Design review of the part built by this model. Coordinates are the model's own, in mm. A direction names the side the tool comes from. Give positions to 0.01 mm unless a question says otherwise; leave off trailing zeros. Loops run counter-clockwise (first coordinate to the right, second up) from the corner with the lowest first, then second, coordinate; pieces in that order, holes last. Notation, with made-up numbers: (58, 44) -> (105, 44) arc R21 cw to (105, 65) -> close; hole circle Ø8 at (-21.5, -21). An arc over 180 degrees is marked (long way). Answer in a Markdown table with one row per item. Add a question column.
(1) Consider section A-A on y = -2.55. Write out the cut boundary in (x, z), then the cut area to 3 significant figures.
(2) Consider section D-D on x = 4.75. Write out the cut boundary in (y, z), then the cut area to 3 significant figures.
(3) Consider section B-B on x = 2.75. Write out the cut boundary in (y, z), then the cut area to 3 significant figures.
(4) Draft analysis for pull direction X (two halves, no side actions). For faces 1 (the cylindrical face through (3.23, -2.339, 6.393)), 2 (the cylindrical face through (5.45, -1.2, 5.58)), 3 (the flat face through (3, -3.15, 1)), 4 (the flat face through (4, -2, 1.55)), state which applies: +X half, -X half, draft (parallel to the pull), parting line (faces both ways), or undercut.
(5) For line 1 (Y direction, x = 5, z = 4.5); line 2 (X direction, y = -1.6, z = 5), list the stretches that pass through material, from the lowest coordinate up.
(6) For faces 5 (the flat face through (0, -2, 4)), 6 (the flat face through (4, -1.55, 4)), list the 3-axis set-ups (+Z, -Z, +X, -X, +Y, -Y) from which the entire face can be reached by the end or side of a thin tool; tool diameter is ignored.
(7) Consider section C-C on z = 3. Write out the cut boundary in (x, y), then the cut area to 3 significant figures.
(8) For pin 1 (0.8 mm diameter, centred on x = 3, y = -2, fed in from +Z); pin 2 (0.5 mm diameter, centred on y = -2.5, z = 3, fed in from +X), all flat-tipped, find the tip position at first contact; note any pin that passes through.
from build123d import *

# Parameters (mm, degrees)
BOSS_EXTRUDE1_DEPTH = 3.15
SHELL1_T            = -1.55
SKETCH2_R           = 2.440449026
CUT_EXTRUDE1_DEPTH  = 1.6


with BuildPart() as part:
    # Sketch1 → Boss-Extrude1 (new body)
    with BuildSketch(Plane(origin=(0, 0, 0), x_dir=(1, 0, 0), z_dir=(0, 1, 0))):
        with BuildLine():
            Line((0, 0), (0, -7.8))
            ThreePointArc((0, -7.8), (5.515432893, -5.515432893), (7.8, 0))
            Line((7.8, 0), (0, 0))
        make_face()
    extrude(amount=-BOSS_EXTRUDE1_DEPTH)

    # Shell1
    shell1_openings = [part.faces().sort_by_distance(p)[0] for p in [
        (3.310422816, -3.15, 3.310422816),
    ]]
    offset(amount=SHELL1_T, openings=shell1_openings, kind=Kind.INTERSECTION)

    # Sketch2 → Cut-Extrude1 (cut)
    with BuildSketch(Plane.XZ.offset(1.55)):
        with Locations((4.030998371, 4.088310158)):
            Circle(SKETCH2_R)
    extrude(amount=CUT_EXTRUDE1_DEPTH, mode=Mode.SUBTRACT)


solid = part.part
Values follow:
| question | item | result |
|---|---|---|
| 1 | outline | (0, 0) -> (7.8, 0) arc R7.8 ccw to (6.45, 4.38) arc R2.44 cw to (5.78, 2.38) arc R6.25 cw to (6.05, 1.55) -> (1.55, 1.55) -> (1.55, 6.05) arc R6.25 cw to (2.3, 5.81) arc R2.44 cw to (4.29, 6.52) arc R7.8 ccw to (0, 7.8) -> close |
| 1 | area | 27.0 mm2 |
| 2 | outline | (-3.15, 0) -> (0, 0) -> (0, 6.19) -> (-1.55, 6.19) -> (-1.55, 1.55) -> (-3.15, 1.55) -> close |
| 2 | area | 12.1 mm2 |
| 3 | outline | (-3.15, 0) -> (0, 0) -> (0, 7.3) -> (-3.15, 7.3) -> (-3.15, 6.17) -> (-1.55, 6.17) -> (-1.55, 1.55) -> (-3.15, 1.55) -> close |
| 3 | area | 15.6 mm2 |
| 4 | face 1 | undercut |
| 4 | face 2 | +X half |
| 4 | face 3 | draft |
| 4 | face 4 | undercut |
| 5 | line 1 | -1.55 to 0 |
| 5 | line 2 | 0 to 1.55 |
| 6 | face 5 | +Z, -Z, -X, +Y, -Y |
| 6 | face 6 | -Y |
| 7 | outline | (0, -3.15) -> (1.55, -3.15) -> (1.55, -1.55) -> (6.22, -1.55) -> (6.22, -3.15) -> (7.2, -3.15) -> (7.2, 0) -> (0, 0) -> close |
| 7 | area | 15.2 mm2 |
| 8 | pin 1 | z = 7.35 |
| 8 | pin 2 | x = 7.3 |
